Geometry check sheet. Reference: the model listing, model coordinates, mm. Coordinates: 2 decimals unless noted, no trailing zeros. Loops run counter-clockwise (first coordinate to the right, second up) from the corner with the lowest first, then second, coordinate; pieces in that order, holes last.
Autodesk Inventor part; units mm, degrees
ref_plane "YZ Plane" through (0, 0, 0) normal (1, 0, 0) x (0, 1, 0)
ref_plane "XZ Plane" through (0, 0, 0) normal (0, 1, 0) x (-1, 0, 0)
ref_plane "XY Plane" through (0, 0, 0) normal (0, 0, 1) x (1, 0, 0)
sketch "Szkic2" plane through (0, 0, 0) normal (0, 0, 1) x (1, 0, 0)
  circle A0 centre (0, 0) radius 16
  dimension "d4" = 32
extrude "Wyciągnięcie proste2" add sketch "Szkic2" along normal blind 460
shell "Skorupa2" thickness 2 removed faces 2 at (4.7224, 2.4785, 0) at (4.7224, 2.4785, 460)
sketch "Szkic3" plane through (0, 0, 0) normal (0, 1, 0) x (-1, 0, 0)
  line L0 (-16, 0) -> (16, 0) construction
  line L1 (0, 0) -> (0, 395.7207) construction
  point P0 (0, 50)
  point P1 (0, 170)
  point P2 (0, 260)
  point P3 (0, 350)
  dimension "d8" = 90
  dimension "d9" = 90
  dimension "d10" = 120
  dimension "d11" = 50
hole "Otwór1" at (0, 0, 50) at (0, 0, 170) at (0, 0, 260) at (0, 0, 350) direction (0, 1, 0) diameter 6 depth 16 tip angle 118
equation "\"PromieńGięcia\" = Grubość"
equation "\"SzerokośćGięciaPodcięcia\" = Grubość"
equation "\"GłębokośćGięciaPodcięcia\" = 0.5 * Grubość"
equation "\"RozmiarPodcięciaNarożnika\" = 4 * Grubość"
equation "\"MinimalnaPozostałość\" = 2 * Grubość"
equation "\"PromieńPrzejścia\" = PromieńGięcia"
equation "\"Rozmiar_promienia_Jacobiego\" = PromieńGięcia"
equation "\"Wielk_odstępu\" = Grubość"
properties part number "Rura_oparcia" material "Aluminium AW-7020"
1) Section check A-A on z = 66.5. Record the cut outline in (x, y).
Data:
outline: circle Ø32 at (0, 0); hole circle Ø28 at (0, 0)
2) Material ranges on probe 1 along Z at (x, y) = (0, 15.1); probe 2 along X at (y, z) = (-1, 272), recorded low to high.
Data:
probe 1: z = 0 to 47, 53 to 167, 173 to 257, 263 to 347, 353 to 460
probe 2: x = -15.97 to -13.96, 13.96 to 15.97
3) Depth check by flat-ended pin: pin 1 (2 mm diameter, centred on x = 4.5, z = 179, fed in from -Y); pin 2 (2 mm diameter, centred on x = 5.5, z = 161.5, fed in from -Y); pin 3 (6 mm diameter, centred on x = 4.5, z = 152, fed in from -Y). Enter the tip coordinate at first touch or a pass-through.
Data:
pin 1: stops at y = -15.61
pin 2: stops at y = -15.35
pin 3: stops at y = -15.93
